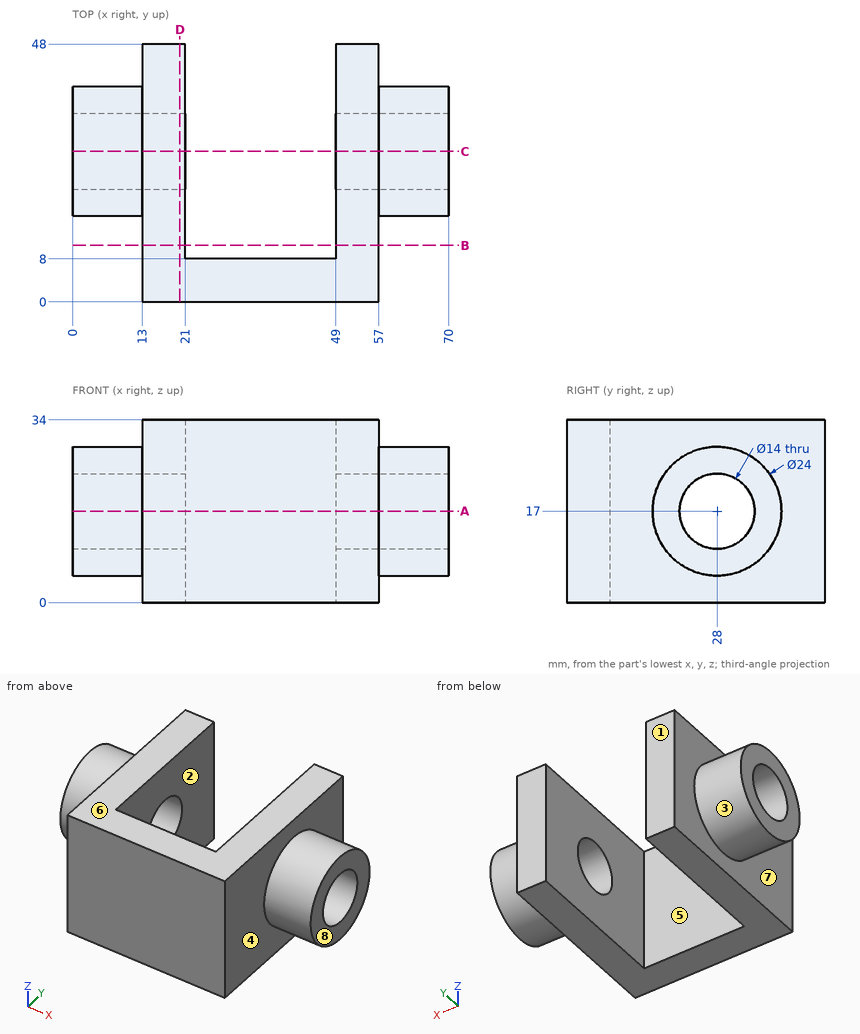
Here's the drawing with two shaded views (mm, measured from the low corner). I have some questions. A direction names the side the tool comes from. Round coordinates to 2 decimals unless told otherwise and drop trailing zeros. Loops run counter-clockwise (first coordinate to the right, second up) from the corner with the lowest first, then second, coordinate; pieces in that order, holes last.
Item 1: Will these pins go through, and if not, where does the flat tip stop? pin 1 Ø3 at (y, z) = (14.5, 5) entering from -X; pin 2 Ø6 at (y, z) = (40.5, 30.5) entering from +X; pin 3 Ø3 at (x, z) = (38.5, 11.5) entering from +Y.
Item 2: If we mould it in two halves opening along X, with no side actions, what happens to the marked faces 5, 6, 7 and 8? For each: +X half, -X half, draft (parallel to the pull), parting line (faces both ways), or undercut.
Item 3: Suppose I cut it at C-C, the plane y = 28. Write out the boundary of the cut face in (x, z), then the cut area to 3 significant figures.
Item 4: Suppose I cut it at A-A, the plane z = 17. Write out the boundary of the cut face in (x, y).
Item 5: Suppose I cut it at B-B, the plane y = 10.5. Write out the boundary of the cut face in (x, z).
Item 6: Suppose I cut it at D-D, the plane x = 20. Write out the boundary of the cut face in (y, z).
Item 7: Which directions (+Z, -Z, +X, -X, +Y, -Y) give clear straight access to the entire face, cutting with the end or side of a thin tool? Please do the marked faces 1, 2, 3 and 4.
Item 8: Please list where these lines run through material, in increasing order: L1, parallel to X at y = 12.5, z = 10.5; L2, parallel to Z at x = 56, y = 28; L3, parallel to Z at x = 11, y = 28.
Reported:
1. pin 1: stops at x = 13
1. pin 2: stops at x = 57
1. pin 3: stops at y = 8
2. face 5: undercut
2. face 6: draft
2. face 7: -X half
2. face 8: +X half
3. outline: (0, 5) - (13, 5) - (13, 0) - (21, 0) - (21, 10) - (0, 10) - close; (0, 24) - (21, 24) - (21, 34) - (13, 34) - (13, 29) - (0, 29) - close; (49, 0) - (57, 0) - (57, 5) - (70, 5) - (70, 10) - (49, 10) - close; (49, 24) - (70, 24) - (70, 29) - (57, 29) - (57, 34) - (49, 34) - close
3. area: 580 mm2
4. outline: (0, 16) - (13, 16) - (13, 0) - (57, 0) - (57, 16) - (70, 16) - (70, 21) - (49, 21) - (49, 8) - (21, 8) - (21, 21) - (0, 21) - close; (0, 35) - (21, 35) - (21, 48) - (13, 48) - (13, 40) - (0, 40) - close; (49, 35) - (70, 35) - (70, 40) - (57, 40) - (57, 48) - (49, 48) - close
5. outline: (13, 0) - (21, 0) - (21, 34) - (13, 34) - close; (49, 0) - (57, 0) - (57, 34) - (49, 34) - close
6. outline: (0, 0) - (48, 0) - (48, 34) - (0, 34) - close; hole circle Ø14 at (28, 17)
7. face 1: +Z, -Z, +X, -X, +Y
7. face 2: +Z, -Z, +Y
7. face 3: -X
7. face 4: +X
8. L1: x = 13 to 21, 49 to 57
8. L2: z = 0 to 10, 24 to 34
8. L3: z = 5 to 10, 24 to 29
